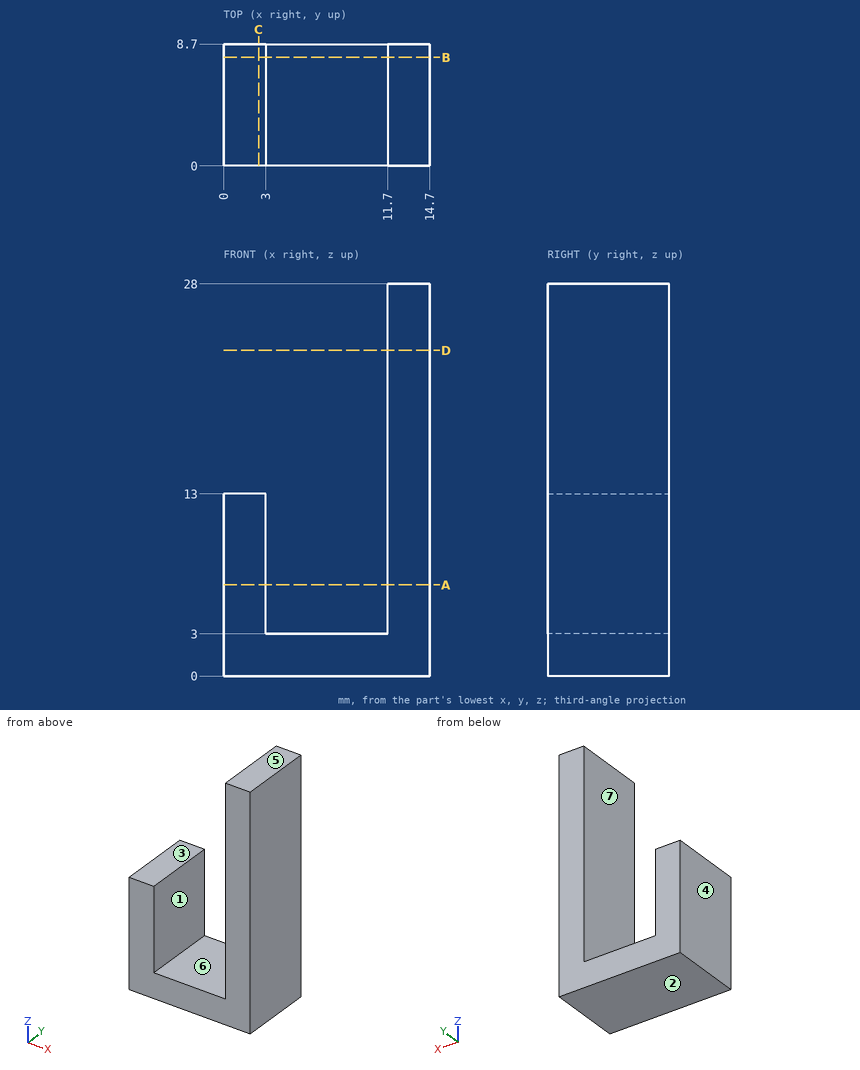
The drawing under review shows one solid part. Ordinate dimensions are in mm from its lowest x, y, z. A direction names the side the tool comes from. Coordinates: 2 decimals unless noted, no trailing zeros. Order: outer loops, then holes, each group sorted by start corner. A loop starts at its lowest first (then second) coordinate and runs counter-clockwise, first axis right, second up. Notation, with made-up numbers: (22, -11.75) -> (39, -11.75) arc R33 ccw to (39, 22.25) -> close; hole circle Ø1 at (-4, -37). An arc over 180 degrees is marked (long way). Use CSV: the item, a comma, the result in double quotes. Start each with the question number.
Item 1: Insertion check: pin 1 (1.5 mm diameter, centred on x = 1.5, y = 5.5, fed in from +Z); pin 2 (4.5 mm diameter, centred on x = 8, y = 3, fed in from +Z). Each pin has a flat end and moves straight along its axis. Give the tip position at first contact, or say it passes through.
Item 2: We need section A-A, the plane z = 6.5. Give the boundary of the cut face in (x, y), then the cut area to 3 significant figures.
Item 3: Draft analysis for pull direction X (two halves, no side actions). For the marked faces 4, 5, 6 and 7, state which applies: pulls with the +X half, pulls with the -X half, needs draft (parallel to the pull), parting line crosses it, or undercut.
Item 4: We need section B-B, the plane y = 7.75. Give the boundary of the cut face in (x, z).
Item 5: We need section D-D, the plane z = 23.25. Give the boundary of the cut face in (x, y), then the cut area to 3 significant figures.
Item 6: For the marked faces 1, 2 and 3, list the 3-axis set-ups (+Z, -Z, +X, -X, +Y, -Y) from which the entire face can be reached by the end or side of a thin tool; tool diameter is ignored.
Item 7: We need section C-C, the plane x = 2.5. Give the boundary of the cut face in (y, z), then the cut area to 3 significant figures.
Item 8: Wall thickness on probe 1 along X at (y, z) = (7.25, 5.5); probe 2 along X at (y, z) = (1.5, 16); probe 3 along Z at (x, y) = (10, 3): over which ranges is each line inside the solid? List them lowest first.
Derived:
1,pin 1,"stops at z = 13"
1,pin 2,"stops at z = 3"
2,outline,"(0, 0) -> (3, 0) -> (3, 8.7) -> (0, 8.7) -> close; (11.7, 0) -> (14.7, 0) -> (14.7, 8.7) -> (11.7, 8.7) -> close"
2,area,"52.2 mm^2"
3,face 4,"pulls with the -X half"
3,face 5,"needs draft"
3,face 6,"undercut"
3,face 7,"undercut"
4,outline,"(0, 0) -> (14.7, 0) -> (14.7, 28) -> (11.7, 28) -> (11.7, 3) -> (3, 3) -> (3, 13) -> (0, 13) -> close"
5,outline,"(11.7, 0) -> (14.7, 0) -> (14.7, 8.7) -> (11.7, 8.7) -> close"
5,area,"26.1 mm^2"
6,face 1,"+Z, +Y, -Y"
6,face 2,"-Z, +X, -X, +Y, -Y"
6,face 3,"+Z, -X, +Y, -Y"
7,outline,"(0, 0) -> (8.7, 0) -> (8.7, 13) -> (0, 13) -> close"
7,area,"113 mm^2"
8,probe 1,"x = 0 to 3, 11.7 to 14.7"
8,probe 2,"x = 11.7 to 14.7"
8,probe 3,"z = 0 to 3"
